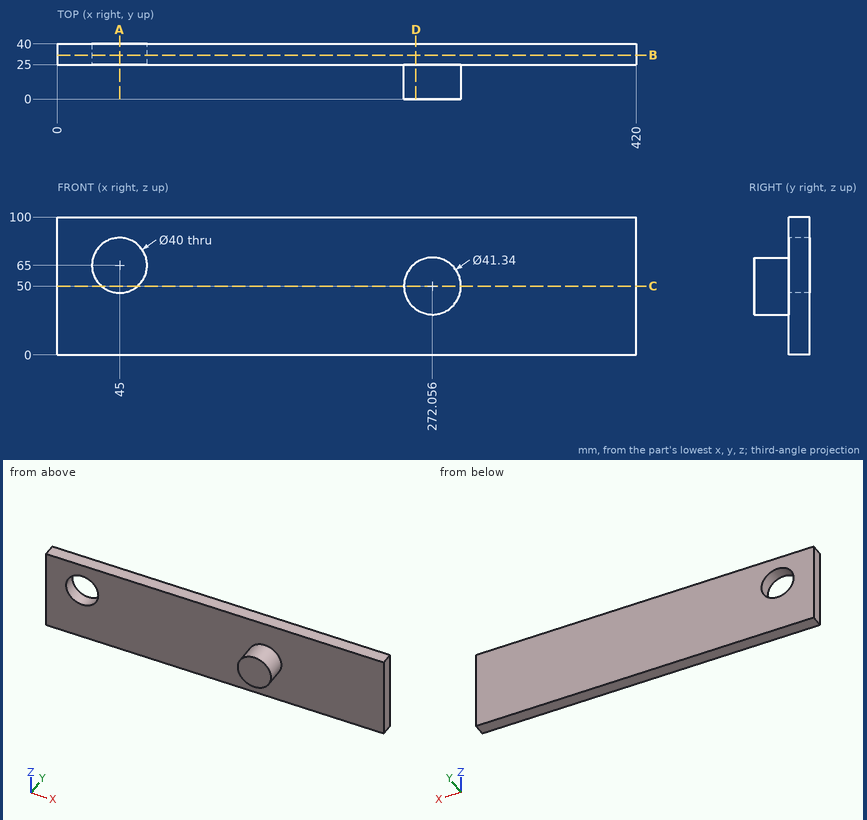
Answer from the drawing. Dimensions are ordinates in mm from the lowest x, y and z of the part. Give positions to 0.01 mm unless a question says otherwise; leave off trailing zeros. Loops run counter-clockwise (first coordinate to the right, second up) from the corner with the lowest first, then second, coordinate; pieces in that order, holes last. Notation, with made-up numbers: (-23, 51.25) - (2, 51.25) arc R5 ccw to (2, 55.25) - close; hole circle Ø2 at (74, 75). An arc over 180 degrees is marked (long way). Answer as CSV lines item,"result". Start each with the question number.
Item 1: Find the intervals of material crossed by line 1 (Z direction, x = 45, y = 33.5); line 2 (Y direction, x = 337, z = 67); line 3 (X direction, y = 24, z = 67) (1 decimal), in increasing order. Write a range as from..to.
Item 2: A cutting plane is placed at A-A on x = 45. Determine the outline of the cut face in (y, z), then the cut area to 3 significant figures.
Item 3: Each of these flat-tipped pins is pushed along its axis until it touches: pin 1 (12 mm diameter, centred on x = 266, y = 11.5, fed in from -Z); pin 2 (10 mm diameter, centred on x = 210, z = 51, fed in from -Y). Where does it stop, or does it pass through?
Item 4: A cutting plane is placed at D-D on x = 260. Determine the outline of the cut face in (y, z), then the cut area to 3 significant figures.
Item 5: A cutting plane is placed at B-B on y = 32. Determine the outline of the cut face in (x, z), then the cut area to 3 significant figures.
Item 6: A cutting plane is placed at C-C on z = 50. Determine the outline of the cut face in (x, y) (1 decimal), then the cut area to 3 significant figures.
Found:
1,line 1,"z = 0..45, 85..100"
1,line 2,"y = 25..40"
1,line 3,"x = 260.3..283.8"
2,outline,"(25, 0) - (40, 0) - (40, 45) - (25, 45) - close; (25, 85) - (40, 85) - (40, 100) - (25, 100) - close"
2,area,"900 mm^2"
3,pin 1,"stops at z = 29.33"
3,pin 2,"stops at y = 25"
4,outline,"(0, 33.21) - (25, 33.21) - (25, 0) - (40, 0) - (40, 100) - (25, 100) - (25, 66.79) - (0, 66.79) - close"
4,area,"2,340 mm^2"
5,outline,"(0, 0) - (420, 0) - (420, 100) - (0, 100) - close; hole circle Ø40 at (45, 65)"
5,area,"40,700 mm^2"
6,outline,"(0, 25) - (31.8, 25) - (31.8, 40) - (0, 40) - close; (58.2, 25) - (251.4, 25) - (251.4, 0) - (292.7, 0) - (292.7, 25) - (420, 25) - (420, 40) - (58.2, 40) - close"
6,area,"6,940 mm^2"
